The model under review builds one solid part; all positions refer to its coordinate system, in mm. Face numbers are marked on the shaded views. Round coordinates to 2 decimals unless told otherwise and drop trailing zeros. Loops run counter-clockwise (first coordinate to the right, second up) from the corner with the lowest first, then second, coordinate; pieces in that order, holes last. Notation, with made-up numbers: M 50.25,75.5 L 73.25,75.5 A12 cw 73.25,98.5 Z; hole C -34,-24 d8. An arc over 180 degrees is marked long. Return JSON: item names as keys, results as strings. Group by question number.
Q1. Consider section D-D (y = -5). State the section outline as (x, z) points.
Q2. Draft analysis for pull direction Y (two halves, no side actions). For the marked faces 1, 2 and 3, state which applies: pulls with the +Y half, pulls with the -Y half, needs draft (parallel to the pull), parting line crosses it, or undercut.
Q3. Clearance check with a flat-ended pin moving along its axis: pin 1 Ø3.5 at (x, y) = (12.7, 0) entering from +Z. State where the tip first meets the part, or that it passes through.
Q4. Consider section C-C (x = 11). State the section outline as (y, z) points, and give its area (3 significant figures).
Q5. To check wall thickness, follow line 1 along Y through (x, z) = (12.7, 1.1); line 2 along Y through (x, z) = (13.75, 1.2); line 3 along X through (y, z) = (-16.5, 0.1). State the ranges of each line that lie inside material, in increasing order.
Q6. Consider section A-A (x = 14.25). State the section outline as (y, z) points, and give its area (3 significant figures).
Q7. Consider section B-B (z = 1.25). State the section outline as (x, y) points.
Autodesk Inventor part; units mm, degrees
ref_plane "YZ Plane" through (0, 0, 0) normal (1, 0, 0) x (0, 1, 0)
ref_plane "XZ Plane" through (0, 0, 0) normal (0, 1, 0) x (-1, 0, 0)
ref_plane "XY Plane" through (0, 0, 0) normal (0, 0, 1) x (1, 0, 0)
sketch "Sketch1" plane through (0, 0, 0) normal (0, 0, 1) x (1, 0, 0)
  circle A0 centre (0, 0) radius 2.1844
  line L0 (0, 0) -> (12.7, 0)
  circle A1 centre (12.7, 0) radius 2.1844
  line L1 (12.7, 0) -> (12.7, -17.78)
  circle A2 centre (12.7, -17.78) radius 2.1844
  circle A3 centre (0, 0) radius 5.08
  circle A4 centre (12.7, 0) radius 5.08
  circle A5 centre (12.7, -17.78) radius 5.08
  line L2 (0, 5.08) -> (12.7, 5.08)
  line L3 (17.78, 0) -> (17.78, -17.78)
  line L4 (-4.5864, -2.1844) -> (8.1136, -19.9644)
  point P0 (-3.5538, -3.63)
  dimension "d8" = 4.3688
  dimension "d9" = 12.7
  dimension "d10" = 4.3688
  dimension "d11" = 17.78
  dimension "d12" = 4.3688
  dimension "d13" = 10.16
  dimension "d14" = 10.16
  dimension "d15" = 10.16
extrude "Extrusion2" add sketch "Sketch1" along normal blind 1.5875 contours A3 L4 | A3 L2 A4 L0 | L0 A4 L1 A5 L4 A3 | A4 L1 A1 L0 | L0 A1 L1 A4 | A3 L4 | A4 L3 A5 L1 | A5
properties part number "Wing poly connection 2"
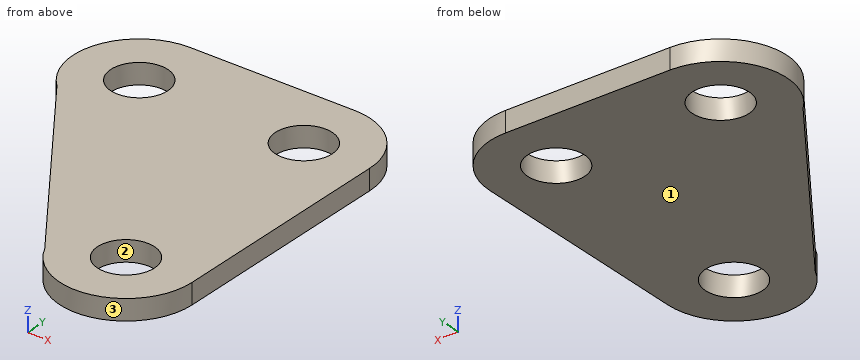
Values:
{
 "1": {"outline": "M -2.58,0 L 17.78,0 L 17.78,1.59 L -2.58,1.59 Z"},
 "2": {"face 1": "needs draft", "face 2": "undercut", "face 3": "pulls with the -Y half"},
 "3": {"pin 1": "passes through"},
 "4": {"outline": "M -22.57,0 L -19.15,0 L -19.15,1.59 L -22.57,1.59 Z; M -16.41,0 L -1.37,0 L -1.37,1.59 L -16.41,1.59 Z; M 1.37,0 L 5.08,0 L 5.08,1.59 L 1.37,1.59 Z", "area": "35.2 mm2"},
 "5": {"line 1": "y = -22.86 to -19.96, -15.6 to -2.18, 2.18 to 5.08", "line 2": "y = -22.75 to -19.7, -15.86 to -1.92, 1.92 to 4.97", "line 3": "x = 5.64 to 10.93, 14.47 to 17.78"},
 "6": {"outline": "M -22.62,0 L -19.32,0 L -19.32,1.59 L -22.62,1.59 Z; M -16.24,0 L -1.54,0 L -1.54,1.59 L -16.24,1.59 Z; M 1.54,0 L 4.84,0 L 4.84,1.59 L 1.54,1.59 Z", "area": "33.8 mm2"},
 "7": {"outline": "M -3.55,-3.63 L 8.11,-19.96 A5.08 ccw 17.78,-17.78 L 17.78,0 A5.08 ccw 12.7,5.08 L 0,5.08 A5.08 ccw Z; hole C 0,0 d4.37; hole C 12.7,-17.78 d4.37; hole C 12.7,0 d4.37"}
}
